Could you check a few things on this model? Use its own coordinates, in mm. Round coordinates to 2 decimals unless told otherwise and drop trailing zeros. Order: outer loops, then holes, each group sorted by start corner. A loop starts at its lowest first (then second) coordinate and runs counter-clockwise, first axis right, second up. Notation, with made-up numbers: (-24.5, -16) - (5.5, -16) arc R26 ccw to (5.5, 16) - close; hole circle Ø10 at (4, 84.25). An arc over 180 degrees is marked (long way). Use one line per item in the form item = value.
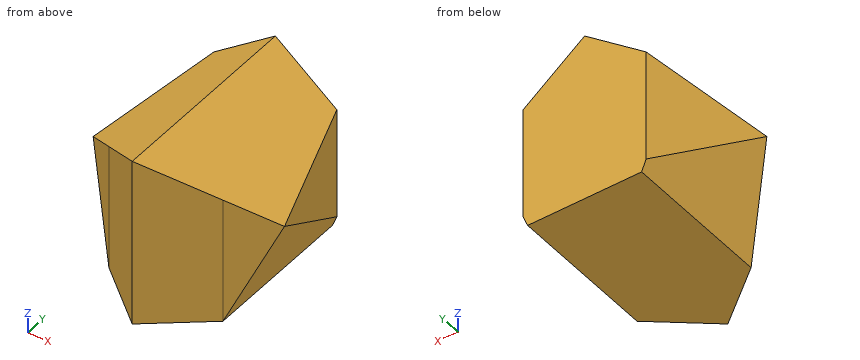
from build123d import *

# Parameters (mm, degrees)
F0_W     = 470
F0_H     = 420
F1_DEPTH = 240
F3_DEPTH = 480.001
F5_DEPTH = 420.001


with BuildPart() as f1:
    # F0 (on Front) → F1 (new body, symmetric)
    with BuildSketch(Plane.XZ):
        Rectangle(F0_W, F0_H)
    extrude(amount=F1_DEPTH, both=True)

    # F2 (on face) → F3 (cut, through all)
    with BuildSketch(Plane.XZ.offset(240)):
        Polygon((0, 210), (235, 30), (235, 210), align=None)
        Polygon((235, 30), (140, -210), (235, -210), align=None)
        Polygon((-235, -210), (-140, -210), (-235, 30), align=None)
        Polygon((-235, 30), (0, 210), (-235, 210), align=None)
    extrude(amount=-F3_DEPTH, mode=Mode.SUBTRACT)

    # F4 (on face) → F5 (cut, through all)
    with BuildSketch(Plane(origin=(0, 0, -210), x_dir=(1, 0, 0), z_dir=(0, 0, -1))):
        Polygon((140, 126.917813), (235, 50.183472), (235, 240), (140, 240), align=None)
        Polygon((0, 240), (140, 126.917813), (140, 240), align=None)
        Polygon((235, 50.183472), (151.042473, -240), (235, -240), align=None)
        Polygon((-235, -240), (-151.042473, -240), (-235, 50.183472), align=None)
        Polygon((-235, 50.183472), (-140, 126.917813), (-140, 240), (-235, 240), align=None)
        Polygon((-140, 126.917813), (0, 240), (-140, 240), align=None)
    extrude(amount=-F5_DEPTH, mode=Mode.SUBTRACT)


solid = f1.part
Item 1: Imagine slicing it at B-B on z = -54. Please give me the cut outline in (x, y), plus the area to 3 significant figures.
Found:
outline = (-201.75, -77.04) - (0, -240) - (201.75, -77.04) - (201.75, 64.74) - (151.04, 240) - (-151.04, 240) - (-201.75, 64.74) - close
area = 152,000 mm2
Item 2: Imagine slicing it at C-C on x = -62. Please give me the cut outline in (y, z), plus the area to 3 significant figures.
Found:
outline = (-189.92, -210) - (240, -210) - (240, 162.51) - (-189.92, 162.51) - close
area = 160,000 mm2
Item 3: Will these pins go through, and if not, where does the flat tip stop? P1, Ø8, axis at x = -173.5, y = 133.5, coming from the +Z side; P2, Ø1.5, axis at y = -4, z = -93.5, coming from the +X side; P3, Ø5, axis at x = 40.5, z = 66.5, coming from the -Y side.
Found:
P1 = 80.17
P2 = 186.41
P3 = -209.31
Item 4: Imagine slicing it at D-D on y = 206. Please give me the cut outline in (x, z), plus the area to 3 significant figures.
Found:
outline = (-160.88, -157.25) - (-140, -210) - (140, -210) - (160.88, -157.25) - (160.88, 86.77) - (0, 210) - (-160.88, 86.77) - close
area = 114,000 mm2
Item 5: Imagine slicing it at A-A on y = 112.5. Please give me the cut outline in (x, z).
Found:
outline = (-187.93, -88.91) - (-140, -210) - (140, -210) - (187.93, -88.91) - (187.93, 66.05) - (0, 210) - (-187.93, 66.05) - close
Item 6: I need wall thicknesses on L1, parallel to Y at x = -140, z = -18; L2, parallel to Y at x = 79, z = 38; L3, parallel to X at y = -214.5, z = -167. Which ranges of each line are inside material? Lowest first, please.
Found:
L1 = -126.92 to 240
L2 = -176.19 to 240
L3 = -31.57 to 31.57
